Check sheet for the drawn part. Datum: minimum x, y, z corner. Units: mm. A direction names the side the tool comes from. Round coordinates to 2 decimals unless told otherwise and drop trailing zeros. Write each loop counter-clockwise with the first axis right and the second up, starting at its lowest first coordinate (ties: lowest second). Pieces come first, ordered by that corner, then holes. Notation, with made-up numbers: M 38.5,-19 L 75.5,-19 A23 ccw 75.5,5 Z; hole C 87,67 d5. An arc over 180 degrees is marked long. One line per item, written item: value.
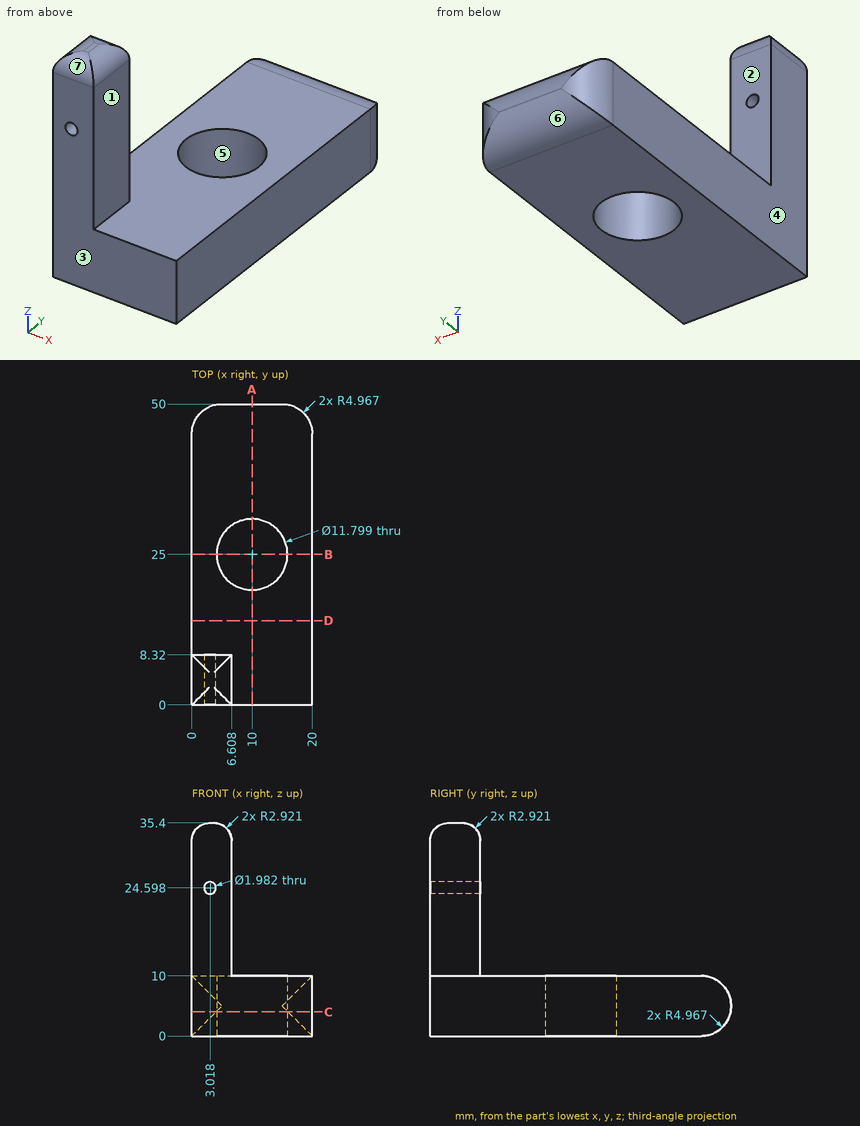
Q1. Scan lines: line 1 (Y direction, x = 6.5, z = 28); line 2 (Z direction, x = 4.25, y = 26.5); line 3 (X direction, y = 20, z = 4.5). Record each from-to range of solid material in increasing order. Write a range as [from, to].
Completed:
line 1: [0, 8.32]
line 2: [0, 10]
line 3: [0, 6.87], [13.13, 20]
Q2. Sectioned sample at C-C on z = 4. Enter the section's corners in (x, y) (1 decimal).
Completed:
outline: M 0,0 L 20,0 L 20,45 A5 ccw 16,49.9 L 4,49.9 A5 ccw 0,45 Z; hole C 10,25 d11.8
Q3. Sectioned sample at D-D on y = 14. Enter the section's corners in (x, z), and give its area (3 significant figures).
Completed:
outline: M 0,0 L 20,0 L 20,10 L 0,10 Z
area: 200 mm^2
Q4. Sectioned sample at A-A on x = 10. Enter the section's corners in (y, z).
Completed:
outline: M 0,0 L 19.1,0 L 19.1,10 L 0,10 Z; M 30.9,0 L 45.03,0 A4.97 ccw 50,4.97 L 50,5.03 A4.97 ccw 45.03,10 L 30.9,10 Z
Q5. Sectioned sample at B-B on y = 25. Enter the section's corners in (x, z).
Completed:
outline: M 0,0 L 4.1,0 L 4.1,10 L 0,10 Z; M 15.9,0 L 20,0 L 20,10 L 15.9,10 Z
Q6. Draft check along Y on the marked faces 4, 5, 6 and 7. Enter one of: pulls with the +Y half, pulls with the -Y half, needs draft (parallel to the pull), parting line crosses it, or undercut.
Completed:
face 4: needs draft
face 5: undercut
face 6: pulls with the +Y half
face 7: pulls with the -Y half
Q7. Depth check by flat-ended pin: P1, Ø4, axis at x = 16.5, y = 13, coming from the +Z side; P2, Ø5.5, axis at x = 2.5, z = 16, coming from the +Y side; P3, Ø3, axis at x = 10, z = 6.5, coming from the +Y side; P4, Ø4, axis at y = 5, z = 23.5, coming from the +X side. Enter the tip coordinate at first touch or a pass-through.
Completed:
P1: z = 10
P2: y = 8.32
P3: y = 50
P4: x = 6.61
Q8. Access from +Z, -Z, +X, -X, +Y, -Y to the whole of each face (thin tool, end or side, straight path). Record for the marked faces 1, 2 and 3.
Completed:
face 1: +Z, +X, +Y, -Y
face 2: +Z, +X, -X, +Y
face 3: +Z, -Z, +X, -X, -Y
